from build123d import *

# Parameters (mm, degrees)
F0_W     = 326
F0_H     = 238
F0_W_2   = 74
F0_H_2   = 110
F0_W_3   = 80
F1_DEPTH = 2
F2_DEPTH = 4
F0_W_4   = 338
F0_H_3   = 250
F3_DEPTH = 40


with BuildPart() as f1:
    # F0 (on Top) → F1 (new body)
    with BuildSketch(Plane.XY):
        with Locations((80, 0)):
            Rectangle(F0_W, F0_H)
        with Locations((-40, -58)):
            Rectangle(F0_W_2, F0_H_2, mode=Mode.SUBTRACT)
        with Locations((40, -58)):
            Rectangle(F0_W_2, F0_H_2, mode=Mode.SUBTRACT)
        with Locations((123, -58)):
            Rectangle(F0_W_3, F0_H_2, mode=Mode.SUBTRACT)
        with Locations((-40, 58)):
            Rectangle(F0_W_2, F0_H_2, mode=Mode.SUBTRACT)
        with Locations((40, 58)):
            Rectangle(F0_W_2, F0_H_2, mode=Mode.SUBTRACT)
        with Locations((123, 58)):
            Rectangle(F0_W_3, F0_H_2, mode=Mode.SUBTRACT)
        with Locations((123, -58)):
            Rectangle(F0_W_3, F0_H_2)
        with Locations((123, 58)):
            Rectangle(F0_W_3, F0_H_2)
        with Locations((40, 58)):
            Rectangle(F0_W_2, F0_H_2)
        with Locations((40, -58)):
            Rectangle(F0_W_2, F0_H_2)
        with Locations((-40, -58)):
            Rectangle(F0_W_2, F0_H_2)
        with Locations((-40, 58)):
            Rectangle(F0_W_2, F0_H_2)
    extrude(amount=F1_DEPTH)

    # F0 (on Top) → F2 (join)
    with BuildSketch(Plane.XY):
        with Locations((123, -58)):
            Rectangle(F0_W_3, F0_H_2)
        with Locations((40, -58)):
            Rectangle(F0_W_2, F0_H_2)
        with Locations((-40, -58)):
            Rectangle(F0_W_2, F0_H_2)
        with Locations((123, 58)):
            Rectangle(F0_W_3, F0_H_2)
        with Locations((40, 58)):
            Rectangle(F0_W_2, F0_H_2)
        with Locations((-40, 58)):
            Rectangle(F0_W_2, F0_H_2)
    extrude(amount=-F2_DEPTH)

    # F0 (on Top) → F3 (join)
    with BuildSketch(Plane.XY):
        with Locations((80, 0)):
            Rectangle(F0_W_4, F0_H_3)
        with Locations((80, 0)):
            Rectangle(F0_W, F0_H, mode=Mode.SUBTRACT)
    extrude(amount=F3_DEPTH)


solid = f1.part
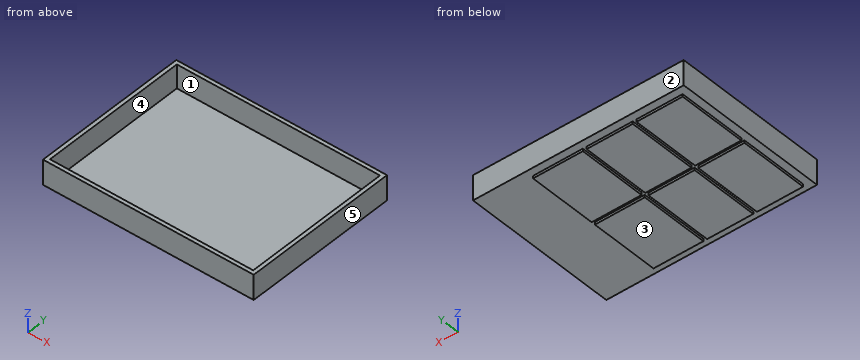
Check sheet for the modelled part. Datum: model origin and axes. Units: mm. Face numbers are marked on the shaded views. A direction names the side the tool comes from. Give positions to 0.01 mm unless a question says otherwise; leave off trailing zeros. Write each loop counter-clockwise with the first axis right and the second up, starting at its lowest first coordinate (ties: lowest second). Pieces come first, ordered by that corner, then holes. Notation, with made-up numbers: (84, -5.5) -> (127, -5.5) arc R37 cw to (127, 30.5) -> close; hole circle Ø6 at (86, 38.5). An arc over 180 degrees is marked (long way). Write item = value, one per line.
Item 1: Sectioned sample at C-C on y = 20. Record the boundary of the cut face in (x, z), and give its area (3 significant figures).
Output:
outline = (-89, 0) -> (-77, 0) -> (-77, -4) -> (-3, -4) -> (-3, 0) -> (3, 0) -> (3, -4) -> (77, -4) -> (77, 0) -> (83, 0) -> (83, -4) -> (163, -4) -> (163, 0) -> (249, 0) -> (249, 40) -> (243, 40) -> (243, 2) -> (-83, 2) -> (-83, 40) -> (-89, 40) -> close
area = 2,040 mm^2
Item 2: Scan lines: probe 1 along Y at (x, z) = (-40.5, 3); probe 2 along X at (y, z) = (-5, 21); probe 3 along Z at (x, y) = (-59, 67). Record each from-to range of solid material in increasing order. Write a range as from..to.
Output:
probe_1 = -125..-119, 119..125
probe_2 = -89..-83, 243..249
probe_3 = -4..2
Item 3: Sectioned sample at B-B on x = 52. Record the boundary of the cut face in (y, z), and give its area (3 significant figures).
Output:
outline = (-125, 0) -> (-113, 0) -> (-113, -4) -> (-3, -4) -> (-3, 0) -> (3, 0) -> (3, -4) -> (113, -4) -> (113, 0) -> (125, 0) -> (125, 40) -> (119, 40) -> (119, 2) -> (-119, 2) -> (-119, 40) -> (-125, 40) -> close
area = 1,840 mm^2
Item 4: Tool access check on the marked faces 1 and 2. Record the directions out of +Z, -Z, +X, -X, +Y, -Y that give a thin tool (end or side, any length) a straight path to the whole face; none if there is none.
Output:
face_1 = +Z
face_2 = +Z, -Z, +X, -X, +Y
Item 5: Release check for a two-part mould opening along X. For the marked faces 3, 4 and 5 record: +X half, -X half, draft (parallel to the pull), parting line (faces both ways), or undercut.
Output:
face_3 = draft
face_4 = undercut
face_5 = +X half
Item 6: Gauge pin test, flat ends, axial feed: pin 1 (12 mm diameter, centred on x = 35.5, y = -39, fed in from +Z); pin 2 (1.2 mm diameter, centred on x = -55.5, z = -3, fed in from +Y); pin 3 (1.2 mm diameter, centred on y = -78.5, z = -1.5, fed in from -X). Record the tip position at first contact, or that the pin passes through.
Output:
pin_1 = 2
pin_2 = 113
pin_3 = -77
Item 7: Sectioned sample at A-A on z = 30.5. Record the boundary of the cut face in (x, y).
Output:
outline = (-89, -125) -> (249, -125) -> (249, 125) -> (-89, 125) -> close; hole (-83, -119) -> (243, -119) -> (243, 119) -> (-83, 119) -> close
